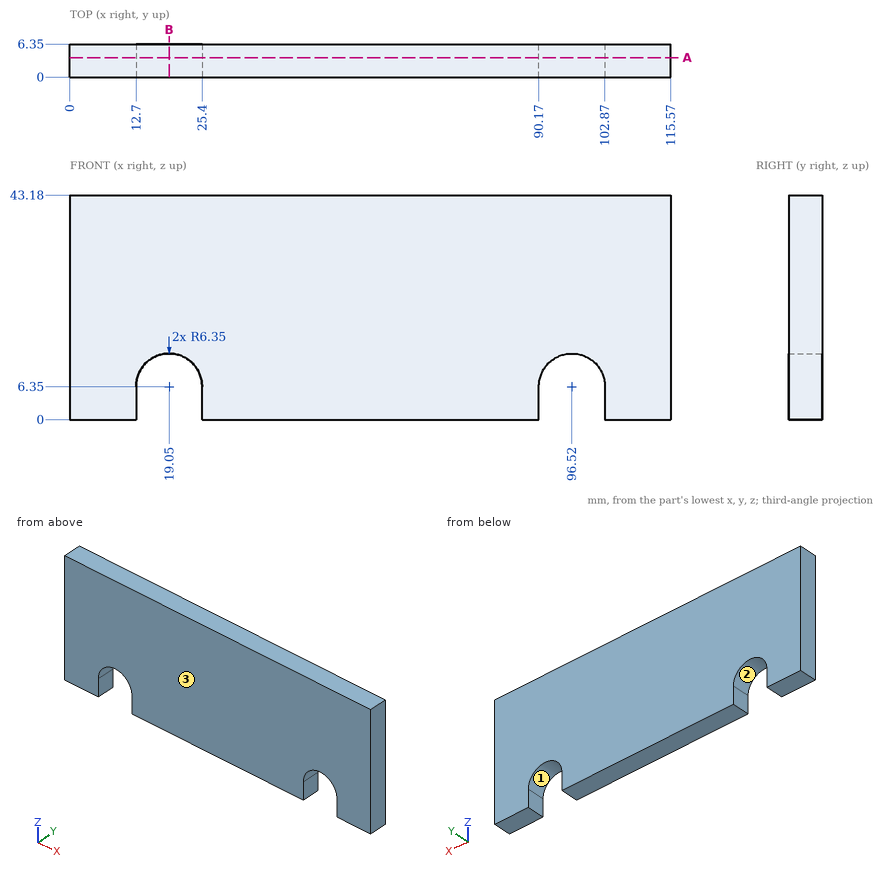
For this review, use the dimensioned drawing (mm, ordinates from the lowest corner) and the shaded views. Round coordinates to 2 decimals unless told otherwise and drop trailing zeros. Order: outer loops, then holes, each group sorted by start corner. A loop starts at its lowest first (then second) coordinate and runs counter-clockwise, first axis right, second up.
1) Consider section A-A (y = 3.75). State the section outline as (x, z) points, plus the area to 3 significant figures.
The answers:
outline: (0, 0) - (12.7, 0) - (12.7, 6.35) arc R6.35 cw to (25.4, 6.35) - (25.4, 0) - (90.17, 0) - (90.17, 6.35) arc R6.35 cw to (102.87, 6.35) - (102.87, 0) - (115.57, 0) - (115.57, 43.18) - (0, 43.18) - close
area: 4,700 mm2
2) Consider section B-B (x = 19.05). State the section outline as (y, z) points, plus the area to 3 significant figures.
The answers:
outline: (0, 12.7) - (6.35, 12.7) - (6.35, 43.18) - (0, 43.18) - close
area: 194 mm2
3) For L1, parallel to X at y = 2.75, z = 11; L2, parallel to X at y = 2.5, z = 12; L3, parallel to Z at x = 21.5, y = 4.25, list the stretches that pass through material, from the lowest coordinate up.
The answers:
L1: x = 0 to 14.73, 23.37 to 92.2, 100.84 to 115.57
L2: x = 0 to 16.15, 21.95 to 93.62, 99.42 to 115.57
L3: z = 12.21 to 43.18
4) Draft analysis for pull direction X (two halves, no side actions). For the marked faces 1, 2 and 3, state which applies: released by +X, released by -X, zero draft, split by the parting line, or undercut.
The answers:
face 1: undercut
face 2: undercut
face 3: zero draft
